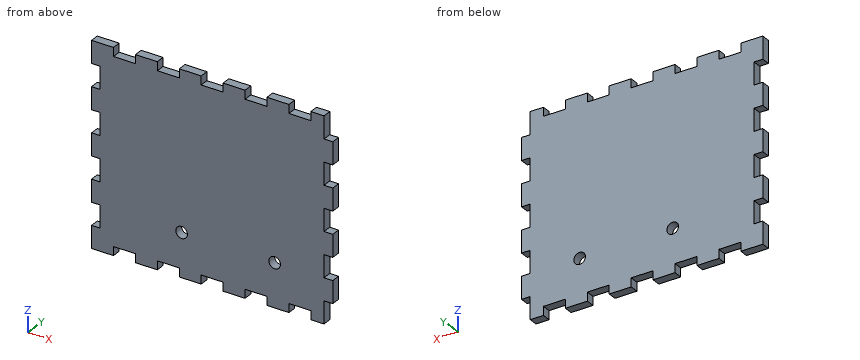
```python
from build123d import *

# Parameters (mm, degrees)
AUFSATZ_LINEAR_AUSTRAGEN1_DEPTH = 3
SKIZZE2_R                       = 2
SCHNITT_LINEAR_AUSTRAGEN1_DEPTH = 3


with BuildPart() as part:
    # Skizze1 → Aufsatz-Linear austragen1 (new body)
    with BuildSketch(Plane(origin=(0, 0, 0), x_dir=(1, 0, 0), z_dir=(0, 1, 0))):
        Polygon((0, 0.000138), (7.544562, 0.000138), (7.544562, 3.000132), (15.090902, 3.000132), (15.090902, 0.000138), (22.635718, 0.000138), (22.635718, 3.000132), (30.18155, 3.000132), (30.18155, 0.000138), (37.726366, 0.000138), (37.726366, 3.000132), (45.272706, 3.000132), (45.272706, 0.000138), (52.81803, 0.000138), (52.81803, 3.000132), (60.36437, 3.000132), (60.36437, 0.000138), (67.90817, 0.000138), (67.90817, 3.000132), (75.45451, 3.000132), (75.45451, 0.000138), (79.99857, 0.000138), (79.99857, 7.666366), (82.99831, 7.666366), (82.99831, 15.332086), (79.99857, 15.332086), (79.99857, 22.99933), (82.99831, 22.99933), (82.99831, 30.665558), (79.99857, 30.665558), (79.99857, 38.333056), (82.99831, 38.333056), (82.99831, 45.99903), (79.99857, 45.99903), (79.99857, 53.666528), (82.99831, 53.666528), (82.99831, 61.332502), (79.99857, 61.332502), (79.99857, 69), (75.45451, 69), (75.45451, 66.000006), (67.90817, 66.000006), (67.90817, 69), (60.36437, 69), (60.36437, 66.000006), (52.81803, 66.000006), (52.81803, 69), (45.272706, 69), (45.272706, 66.000006), (37.726366, 66.000006), (37.726366, 69), (30.18155, 69), (30.18155, 66.000006), (22.635718, 66.000006), (22.635718, 69), (15.090902, 69), (15.090902, 66.000006), (7.544562, 66.000006), (7.544562, 69), (0, 69), (0, 61.332502), (2.99974, 61.332502), (2.99974, 53.666528), (0, 53.666528), (0, 45.99903), (2.99974, 45.99903), (2.99974, 38.333056), (0, 38.333056), (0, 30.665558), (2.99974, 30.665558), (2.99974, 22.99933), (0, 22.99933), (0, 15.332086), (2.99974, 15.332086), (2.99974, 7.666366), (0, 7.666366), align=None)
    extrude(amount=AUFSATZ_LINEAR_AUSTRAGEN1_DEPTH)

    # Skizze2 → Schnitt-Linear austragen1 (cut)
    with BuildSketch(Plane.XZ):
        with Locations((62.99857, -54.000006)):
            Circle(SKIZZE2_R)
        with Locations((30.99857, -54.000006)):
            Circle(SKIZZE2_R)
    extrude(amount=-SCHNITT_LINEAR_AUSTRAGEN1_DEPTH, mode=Mode.SUBTRACT)


solid = part.part
```
For this review, take the finished solid that the model builds, in its own axes (mm). Give positions to 0.01 mm unless a question says otherwise; leave off trailing zeros. Write each loop counter-clockwise with the first axis right and the second up, starting at its lowest first coordinate (ties: lowest second). Pieces come first, ordered by that corner, then holes. Notation, with made-up numbers: M 56,11 L 115,11 A23 cw 115,25 Z; hole C 73.25,49.5 d8. An arc over 180 degrees is marked long. One line per item, written item: value.
1) For line 1 (X direction, y = 1.8, z = -59); line 2 (Z direction, x = 56, y = 2.4); line 3 (X direction, y = 2.7, z = -52.5), list the stretches that pass through material, from the lowest coordinate up. Write a range as from..to.
Results are:
line 1: x = 3..83
line 2: z = -66..-3
line 3: x = 0..29.68, 32.32..61.68, 64.32..80
2) Take a section at C-C, the plane z = -58.5. Write out the cut boundary in (x, y).
Results are:
outline: M 3,0 L 83,0 L 83,3 L 3,3 Z
3) Take a section at B-B, the plane x = 69. Write out the cut boundary in (y, z).
Results are:
outline: M 0,-66 L 3,-66 L 3,-3 L 0,-3 Z
4) Take a section at A-A, the plane y = 0.6. Count the separate pieces of the cut face and the enclosed holes in it, then the cut area to 3 significant figures.
Results are:
separate pieces: 1
enclosed holes: 2
area: 5,270 mm²
5) For P1, Ø0.9, axis at y = 1, z = -67, coming from the +X side; P2, Ø0.9, axis at x = 82, y = 2, coming from the +Z side; P3, Ø1.5, axis at x = 26.5, y = 1.5, coming from the -Z side, all flat-tipped, find the tip position at first contact; note any pin that passes through.
Results are:
P1: stops at x = 80
P2: stops at z = -7.67
P3: stops at z = -66
